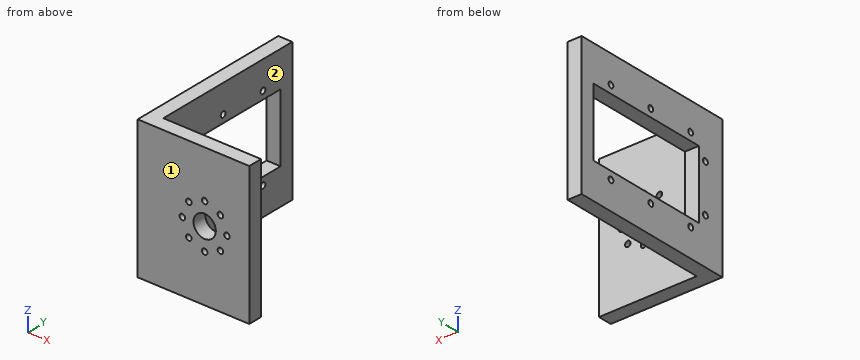
from build123d import *

# Parameters (mm, degrees)
SKETCH1_W           = 40
SKETCH1_H           = 50
SKETCH1_R           = 4
SKETCH1_R_2         = 1
BOSS_EXTRUDE1_DEPTH = 5
SKETCH3_W           = 5
SKETCH3_H           = 50
BOSS_EXTRUDE2_DEPTH = 60
SKETCH4_R           = 1.025
SKETCH4_W           = 24.4
SKETCH4_H           = 45
CUT_EXTRUDE1_DEPTH  = 41


with BuildPart() as part:
    # Sketch1 → Boss-Extrude1 (new body)
    with BuildSketch(Plane(origin=(0, 0, 0), x_dir=(1, 0, 0), z_dir=(0, 1, 0))):
        with Locations((20, 25)):
            Rectangle(SKETCH1_W, SKETCH1_H)
        with Locations((24, 25)):
            Circle(SKETCH1_R, mode=Mode.SUBTRACT)
        with Locations((24, 33)):
            Circle(SKETCH1_R_2, mode=Mode.SUBTRACT)
        with Locations((29.656854249, 30.656854249)):
            Circle(SKETCH1_R_2, mode=Mode.SUBTRACT)
        with Locations((32, 25)):
            Circle(SKETCH1_R_2, mode=Mode.SUBTRACT)
        with Locations((29.656854249, 19.343145751)):
            Circle(SKETCH1_R_2, mode=Mode.SUBTRACT)
        with Locations((24, 17)):
            Circle(SKETCH1_R_2, mode=Mode.SUBTRACT)
        with Locations((18.343145751, 19.343145751)):
            Circle(SKETCH1_R_2, mode=Mode.SUBTRACT)
        with Locations((16, 25)):
            Circle(SKETCH1_R_2, mode=Mode.SUBTRACT)
        with Locations((18.343145751, 30.656854249)):
            Circle(SKETCH1_R_2, mode=Mode.SUBTRACT)
    extrude(amount=BOSS_EXTRUDE1_DEPTH)

    # Sketch3 → Boss-Extrude2 (add)
    with BuildSketch(Plane(origin=(0, 0, 0), x_dir=(1, 0, 0), z_dir=(0, 1, 0))):
        with Locations((2.5, 25)):
            Rectangle(SKETCH3_W, SKETCH3_H)
    extrude(amount=BOSS_EXTRUDE2_DEPTH)

    # Sketch4 → Cut-Extrude1 (cut, through all)
    with BuildSketch(Plane.ZY):
        with Locations((-40, 47.5)):
            Circle(SKETCH4_R)
        with Locations((-10, 47.5)):
            Circle(SKETCH4_R)
        with Locations((-40, 30.5)):
            Circle(SKETCH4_R)
        with Locations((-10, 30.5)):
            Circle(SKETCH4_R)
        with Locations((-40, 13.5)):
            Circle(SKETCH4_R)
        with Locations((-33.5, 7.2)):
            Circle(SKETCH4_R)
        with Locations((-16.5, 7.2)):
            Circle(SKETCH4_R)
        with Locations((-10, 13.5)):
            Circle(SKETCH4_R)
        with Locations((-25, 32.5)):
            Rectangle(SKETCH4_W, SKETCH4_H)
    extrude(amount=-CUT_EXTRUDE1_DEPTH, mode=Mode.SUBTRACT)


solid = part.part
Verification items for the finished model (mm, model axes). Face numbers are marked on the shaded views. A direction names the side the tool comes from. Round coordinates to 2 decimals unless told otherwise and drop trailing zeros. Order: outer loops, then holes, each group sorted by start corner. A loop starts at its lowest first (then second) coordinate and runs counter-clockwise, first axis right, second up.
1. Go/stop test with flat-tipped pins: P1, Ø2.5, axis at x = 29.66, z = -19.34, coming from the +Y side; P2, Ø1.5, axis at x = 29, z = -5.5, coming from the -Y side. Record where each tip stops, or that it passes through.
Final values:
P1: stops at y = 5
P2: stops at y = 0
2. Section check B-B on y = 30.5. Record the cut outline in (x, z) (3 decimals), then the cut area to 4 significant figures.
Final values:
outline: (0, -50) - (5, -50) - (5, -41.025) - (0, -41.025) - close; (0, -38.975) - (5, -38.975) - (5, -37.2) - (0, -37.2) - close; (0, -12.8) - (5, -12.8) - (5, -11.025) - (0, -11.025) - close; (0, -8.975) - (5, -8.975) - (5, 0) - (0, 0) - close
area: 107.5 mm2
3. Section check C-C on z = -25. Record the cut outline in (x, y), then the cut area to 3 significant figures.
Final values:
outline: (0, 0) - (15, 0) - (15, 5) - (5, 5) - (5, 10) - (0, 10) - close; (0, 55) - (5, 55) - (5, 60) - (0, 60) - close; (17, 0) - (20, 0) - (20, 5) - (17, 5) - close; (28, 0) - (31, 0) - (31, 5) - (28, 5) - close; (33, 0) - (40, 0) - (40, 5) - (33, 5) - close
area: 190 mm2
4. Section check A-A on x = 24. Record the cut outline in (y, z).
Final values:
outline: (0, -50) - (5, -50) - (5, -34) - (0, -34) - close; (0, -32) - (5, -32) - (5, -29) - (0, -29) - close; (0, -21) - (5, -21) - (5, -18) - (0, -18) - close; (0, -16) - (5, -16) - (5, 0) - (0, 0) - close
5. Access from +Z, -Z, +X, -X, +Y, -Y to the whole of each face (thin tool, end or side, straight path). Record for the marked faces 1 and 2.
Final values:
face 1: +Z, -Z, +X, -X, -Y
face 2: +Z, -Z, +X, +Y
6. Thickness scan on L1, parallel to Y at x = 2, z = -10 (3 decimals); L2, parallel to Z at x = 24, y = 2; L3, parallel to Z at x = 16, y = 3. Record the ranges inside material, lowest first.
Final values:
L1: y = 0 to 12.475, 14.525 to 29.475, 31.525 to 46.475, 48.525 to 60
L2: z = -50 to -34, -32 to -29, -21 to -18, -16 to 0
L3: z = -50 to -26, -24 to 0
7. Section check D-D on y = 17. Record the cut outline in (x, z).
Final values:
outline: (0, -50) - (5, -50) - (5, -37.2) - (0, -37.2) - close; (0, -12.8) - (5, -12.8) - (5, 0) - (0, 0) - close
